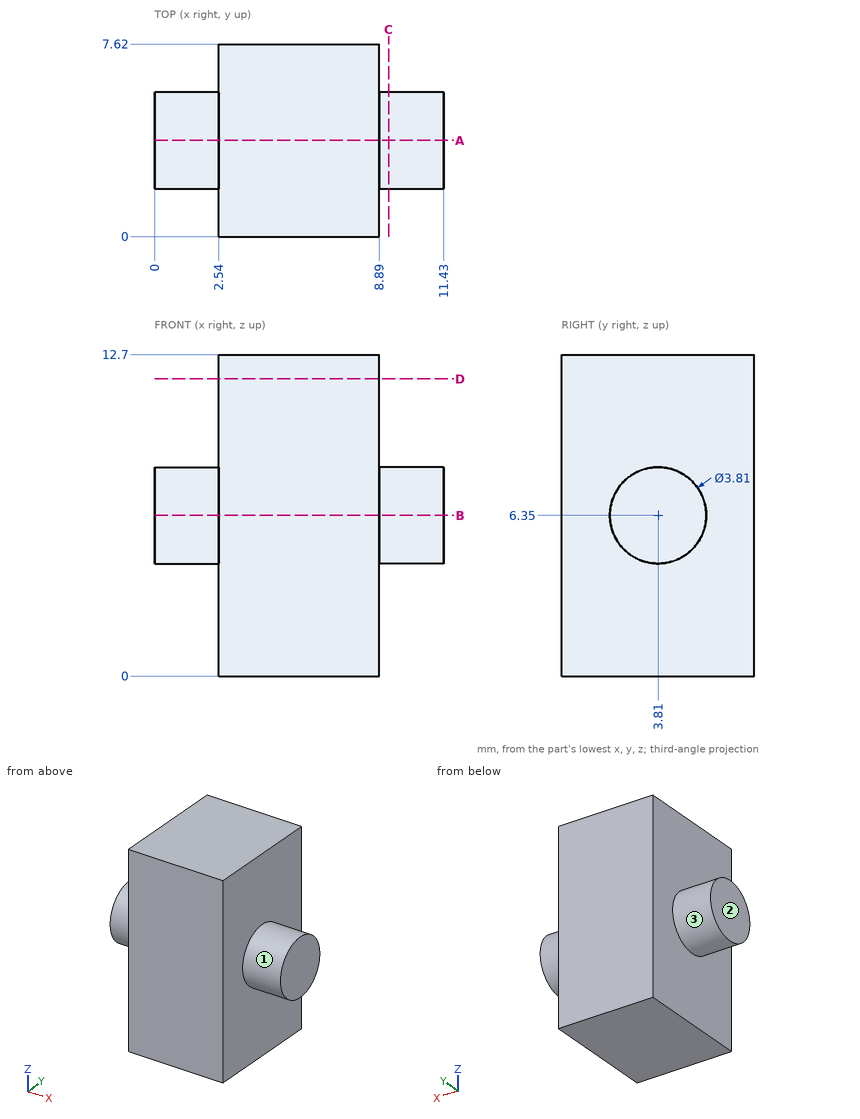
The figure shows three views and two pictorial views of one solid part (mm, origin at its lowest corner). Answer the questions. A direction names the side the tool comes from. Round coordinates to 2 decimals unless told otherwise and drop trailing zeros. Write each loop counter-clockwise with the first axis right and the second up, starting at its lowest first coordinate (ties: lowest second). Pieces come first, ordered by that corner, then holes. Notation, with made-up numbers: (-11.5, 77.25) - (0.5, 77.25) arc R23 ccw to (0.5, 113.25) - close; hole circle Ø2 at (80.25, 67). An arc over 180 degrees is marked (long way). One line per question, with ' | ' between items. Start each with the question number.
1. For the marked faces 1, 2 and 3, determine the directions among +Z, -Z, +X, -X, +Y, -Y from which every point of the face is accessible in a straight line to the end or side of a thin tool.
2. Section D-D (z = 11.75) is taken. Determine the outline of the cut face in (x, y), and give its area (3 significant figures).
3. Section C-C (x = 9.25) is taken. Determine the outline of the cut face in (y, z) (3 decimals).
4. Section B-B (z = 6.35) is taken. Determine the outline of the cut face in (x, y) (3 decimals).
5. Section A-A (y = 3.81) is taken. Determine the outline of the cut face in (x, z) (3 decimals), and give its area (4 significant figures).
6. Find the intervals of material crossed by probe 1 along X at (y, z) = (3.25, 12); probe 2 along Y at (x, z) = (1.25, 7); probe 3 along Z at (x, y) = (10.25, 2.5), in increasing order. Write a range as [from, to].
Filled in:
1) face 1: +X | face 2: +Z, -Z, -X, +Y, -Y | face 3: -X
2) outline: (2.54, 0) - (8.89, 0) - (8.89, 7.62) - (2.54, 7.62) - close | area: 48.4 mm²
3) outline: circle Ø3.81 at (3.81, 6.35)
4) outline: (0, 1.905) - (2.54, 1.905) - (2.54, 0) - (8.89, 0) - (8.89, 1.905) - (11.43, 1.905) - (11.43, 5.715) - (8.89, 5.715) - (8.89, 7.62) - (2.54, 7.62) - (2.54, 5.715) - (0, 5.715) - close
5) outline: (0, 4.445) - (2.54, 4.445) - (2.54, 0) - (8.89, 0) - (8.89, 4.445) - (11.43, 4.445) - (11.43, 8.255) - (8.89, 8.255) - (8.89, 12.7) - (2.54, 12.7) - (2.54, 8.255) - (0, 8.255) - close | area: 100.0 mm²
6) probe 1: [2.54, 8.89] | probe 2: [2.02, 5.6] | probe 3: [4.97, 7.73]
